Design review of the part built by this model. Coordinates are the model's own, in mm. A direction names the side the tool comes from. Give positions to 0.01 mm unless a question says otherwise; leave off trailing zeros. Loops run counter-clockwise (first coordinate to the right, second up) from the corner with the lowest first, then second, coordinate; pieces in that order, holes last. Notation, with made-up numbers: (56, 56) - (99, 56) arc R13 cw to (99, 63) - close; hole circle Ø11 at (6, 88.25). An arc over 180 degrees is marked (long way). One line per item, written item: value. Start each with the question number.
```python
from build123d import *

# Parameters (mm, degrees)
SKETCH010_R         = 3.2
PAD003_DEPTH        = 12
HOLE004_D           = 6.6
HOLE004_DEPTH       = 25
HOLE004_CBORE_D     = 9
HOLE004_CBORE_DEPTH = 6.1
HOLE005_D           = 3.4
HOLE005_DEPTH       = 10
HOLE005_CBORE_D     = 4.6
HOLE005_CBORE_DEPTH = 5
HOLE005_TIPS_R      = 1.7
HOLE006_D           = 3.4
HOLE006_DEPTH       = 10
HOLE006_CBORE_D     = 4.6
HOLE006_CBORE_DEPTH = 5


with BuildPart() as part:
    # Sketch010 (on DatumPlane) → Pad003 (new body)
    with BuildSketch(Plane.XZ.offset(20)):
        Polygon((30, -11.819805), (30, -26.464466), (26.464466, -30), (13, -30), (10, -33), (-10, -33), (-13, -30), (-26.464466, -30), (-30, -26.464466), (-30, -11.819805), (-26.464466, -8.284271), (-20, -8.284271), (-8.284271, -20), (8.284271, -20), (20, -8.284271), (26.464466, -8.284271), align=None)
        with Locations((20, -20)):
            Circle(SKETCH010_R, mode=Mode.SUBTRACT)
        with Locations((-20, -20)):
            Circle(SKETCH010_R, mode=Mode.SUBTRACT)
    extrude(amount=PAD003_DEPTH)

    # Hole004
    with Locations(Plane.XY.offset(-20)):
        with Locations((0, -26)):
            CounterBoreHole(HOLE004_D / 2, HOLE004_CBORE_D / 2, HOLE004_CBORE_DEPTH, depth=HOLE004_DEPTH)

    # Hole005
    with Locations(Plane.YZ.offset(30)):
        with Locations((-26, -20)):
            CounterBoreHole(HOLE005_D / 2, HOLE005_CBORE_D / 2, HOLE005_CBORE_DEPTH, depth=HOLE005_DEPTH)

    # Hole005 tips → Hole005 tip 1 section 0
    with BuildSketch(Plane.YZ.offset(20), mode=Mode.PRIVATE) as hole005_tip_1_s0:
        with Locations((-26, -20)):
            Circle(HOLE005_TIPS_R)
    loft([hole005_tip_1_s0.sketch, Vertex(18.978537, -26, -20)], mode=Mode.SUBTRACT)

    # Hole006
    with Locations(Plane(origin=(-30, 0, 0), x_dir=(0, 1, 0), z_dir=(-1, 0, 0))):
        with Locations((-26, 20)):
            CounterBoreHole(HOLE006_D / 2, HOLE006_CBORE_D / 2, HOLE006_CBORE_DEPTH, depth=HOLE006_DEPTH)


solid = part.part
```
(1) Take a section at C-C on z = -14.75. State the section outline as (x, y) points.
(2) Take a section at D-D on z = -29. State the section outline as (x, y) points, and give its area (3 significant figures).
(3) Machinability: for faces 5 (the cylindrical face through (2.419, -22.206, -23.007)), 6 (the flat face through (-20, -26, -30)), 7 (the flat face through (20, -26, -30)), 8 (the flat face through (25, -26, -22)), which of the approach directions +Z, -Z, +X, -X, +Y, -Y give a long, thin tool a straight path to every point of the face, cutting with its end or side? Answer none if there is none.
(4) For pin 1 Ø7 at (x, y) = (-2, -24.5) entering from +Z; pin 2 Ø3 at (y, z) = (-26, -20) entering from +X; pin 3 Ø1.5 at (x, y) = (-17, -25) entering from -Z; pin 4 Ø1.5 at (x, z) = (20, -20.5) entering from -Y, all flat-tipped, find the tip position at first contact; note any pin that passes through.
(5) Take a section at A-A on x = 0. State the section outline as (y, z) points.
(6) To check wall thickness, follow L1, parallel to Y at x = -26.1, z = -20; L2, parallel to X at y = -20.25, z = -22; L3, parallel to Y at x = 24.05, z = -20. State the ranges of each line that lie inside material, in increasing order. Write a range as from..to.
(7) Draft analysis for pull direction Y (two halves, no side actions). For faces 1 (the cylindrical face through (27.535, -26.499, -22.245)), 2 (the flat face through (0.4, -32, -20.5)), 3 (the flat face through (0.4, -20, -20.5)), 4 (the flat face through (28.21, -25.92, -10.03)), state which applies: pulls with the +Y half, pulls with the -Y half, needs draft (parallel to the pull), parting line crosses it, or undercut.
(8) Take a section at B-B on z = -10.25. State the section outline as (x, y) points.
Here are the results:
1. outline: (-30, -32) - (-13.53, -32) - (-13.53, -20) - (-30, -20) - close; (13.53, -32) - (30, -32) - (30, -20) - (13.53, -20) - close
2. outline: (-27.46, -32) - (27.46, -32) - (27.46, -20) - (-27.46, -20) - close; hole circle Ø6.6 at (0, -26)
2. area: 625 mm²
3. face 5: +Z
3. face 6: -Z, -X, +Y, -Y
3. face 7: -Z, +X, +Y, -Y
3. face 8: +X
4. pin 1: z = -20
4. pin 2: x = 17.17
4. pin 3: z = -30
4. pin 4: through
5. outline: (-32, -33) - (-29.3, -33) - (-29.3, -26.1) - (-30.5, -26.1) - (-30.5, -20) - (-32, -20) - close; (-22.7, -33) - (-20, -33) - (-20, -20) - (-21.5, -20) - (-21.5, -26.1) - (-22.7, -26.1) - close
6. L1: -32..-28.3, -23.7..-20
6. L2: -30..-22.5, -17.5..17.5, 22.5..30
6. L3: -32..-27.7, -24.3..-20
7. face 1: undercut
7. face 2: pulls with the -Y half
7. face 3: pulls with the +Y half
7. face 4: needs draft
8. outline: (-28.43, -32) - (-18.03, -32) - (-18.03, -20) - (-28.43, -20) - close; (18.03, -32) - (28.43, -32) - (28.43, -20) - (18.03, -20) - close
